Input: part model. Units: mm. Frame: model coordinates. Face numbers are marked on the shaded views. A direction names the side the tool comes from. Round coordinates to 2 decimals unless told otherwise and drop trailing zeros. Write each loop counter-clockwise with the first axis right and the second up, starting at its lowest first coordinate (ties: lowest second). Pieces come first, ordered by that corner, then holes. Notation, with made-up numbers: (4, -32) - (20, -32) arc R19 ccw to (20, -28) - close; hole circle Ø10 at (-31.5, 47). An arc over 180 degrees is marked (long way). One line per item, written item: value. Start each with the question number.
```python
from build123d import *

# Parameters (mm, degrees)
BOSS_EXTRUDE1_DEPTH = 6.35
SKETCH2_R           = 2.286
CUT_EXTRUDE1_DEPTH  = 101.585266767


with BuildPart() as part:
    # Sketch1 → Boss-Extrude1 (new body)
    with BuildSketch(Plane(origin=(0, 0, 0), x_dir=(1, 0, 0), z_dir=(0, 1, 0))):
        Polygon((21.229343583, -21.824581583), (29.62595728, -24.897159466), (70.66112252, -24.897159466), (70.66112252, -61.327405263), (48.489495365, -61.327405263), (21.229343583, -71.302728943), (17.95612252, -62.357805865), (30.65612252, -57.710487253), (30.65612252, -35.416823273), (17.95612252, -30.769504661), align=None)
    extrude(amount=BOSS_EXTRUDE1_DEPTH)

    # Sketch2 → Cut-Extrude1 (cut, through all)
    with BuildSketch(Plane(origin=(0, 6.35, 0), x_dir=(1, 0, 0), z_dir=(0, 1, 0))):
        with Locations(Location((24.30612252, -65.105493971, 0), (0, 0, 270))):
            Circle(SKETCH2_R)
        with Locations(Location((24.30612252, -28.021816555, 0), (0, 0, 270))):
            Circle(SKETCH2_R)
    extrude(amount=-CUT_EXTRUDE1_DEPTH, mode=Mode.SUBTRACT)


solid = part.part
```
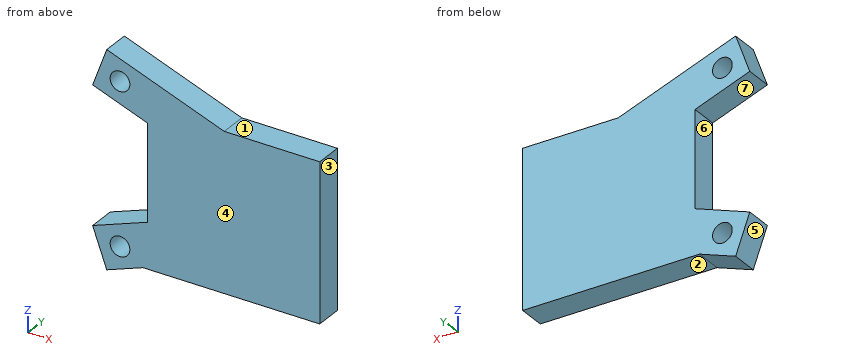
Q1. Cut plane B-B, the plane z = 28.5. Output: boundary loops of the cut face in (x, y), and give its area (3 significant figures).
Q2. Access query for the marked faces 1, 2 and 3. Directions: +Z, -Z, +X, -X, +Y, -Y. A direction counts if a zero-diameter tool reaches every point of the face in a straight line with its end or side. Return the directions, or none.
Q3. Cut plane A-A, the plane x = 23.5. Output: boundary loops of the cut face in (y, z), and give its area (3 significant figures).
Q4. Pull-direction query (Z, two-part tool) for the marked faces 4, 5, 6 and 7; classes: pulls with the +Z half, pulls with the -Z half, needs draft (parallel to the pull), parting line crosses it, or undercut.
Q5. Cut plane C-C, the plane y = 5.25. Output: boundary loops of the cut face in (x, z).
Q6. Material intervals for probe 1 along Z at (x, y) = (22.5, 5.75); probe 2 along Z at (x, y) = (51, 2.5); probe 3 along Z at (x, y) = (21.5, 1.75), sorted ascending. Write a range as from..to.
Q7. Contact query for flat-ended pins moving along their axis: pin 1 Ø1.9 at (y, z) = (2, 49.5) entering from -X; pin 2 Ø1.5 at (x, y) = (38, 2) entering from +Z; pin 3 Ø1 at (x, y) = (29, 5) entering from -Z; pin 4 Ø2.5 at (x, z) = (24.31, 28.02) entering from -Y. Output: stop coordinate, or through.
Q8. Cut plane D-D, the plane z = 66.5. Output: boundary loops of the cut face in (x, y).
A:
1. outline: (18.79, 0) - (22.07, 0) - (22.07, 6.35) - (18.79, 6.35) - close; (26.54, 0) - (70.66, 0) - (70.66, 6.35) - (26.54, 6.35) - close
1. area: 301 mm²
2. face 1: +Z, +X, +Y, -Y
2. face 2: -Z, +X, +Y, -Y
2. face 3: +Z, -Z, +X, +Y, -Y
3. outline: (0, 22.66) - (6.35, 22.66) - (6.35, 25.88) - (0, 25.88) - close; (0, 30.16) - (6.35, 30.16) - (6.35, 32.8) - (0, 32.8) - close; (0, 60.33) - (6.35, 60.33) - (6.35, 62.97) - (0, 62.97) - close; (0, 67.24) - (6.35, 67.24) - (6.35, 70.47) - (0, 70.47) - close
3. area: 74.5 mm²
4. face 4: needs draft
4. face 5: pulls with the -Z half
4. face 6: undercut
4. face 7: undercut
5. outline: (17.96, 30.77) - (21.23, 21.82) - (29.63, 24.9) - (70.66, 24.9) - (70.66, 61.33) - (48.49, 61.33) - (21.23, 71.3) - (17.96, 62.36) - (30.66, 57.71) - (30.66, 35.42) - close; hole circle Ø4.57 at (24.31, 28.02); hole circle Ø4.57 at (24.31, 65.11)
6. probe 1: z = 22.29..26.62, 29.42..32.43, 60.7..63.7, 66.51..70.84
6. probe 2: z = 24.9..61.33
6. probe 3: z = 21.92..32.07, 61.06..71.2
7. pin 1: stops at x = 30.66
7. pin 2: stops at z = 65.44
7. pin 3: stops at z = 24.49
7. pin 4: passes through
8. outline: (19.47, 0) - (22.49, 0) - (22.49, 6.35) - (19.47, 6.35) - close; (26.12, 0) - (34.35, 0) - (34.35, 6.35) - (26.12, 6.35) - close
